Part print with two shaded views. Sizes in mm from the minimum x, y, z corner. A direction names the side the tool comes from. Round coordinates to 2 decimals unless told otherwise and drop trailing zeros. Write each loop counter-clockwise with the first axis right and the second up, starting at its lowest first coordinate (ties: lowest second). Pieces come first, ordered by that corner, then holes. Notation, with made-up numbers: (86, -22) -> (105, -22) arc R22 ccw to (105, 3) -> close; hole circle Ø11 at (15.5, -2.75). An arc over 180 degrees is marked (long way). Return JSON: item names as keys, results as strings. Group by question number.
(1) Tool access for the marked faces 1, 2 and 3: list every direction of +Z, -Z, +X, -X, +Y, -Y with a clear straight run to the whole face (end or side of a thin tool).
(2) Drill centre lines: L1, parallel to Z at x = 69.5, y = 12; L2, parallel to Y at x = 11, z = 58.5; L3, parallel to Y at x = 35, z = 49. Where is each one in solid material? Low to high. Write a range as from..to.
(3) Saw through at C-C (y = 36). List the corners of the cut face in (x, z), plus the area to 3 significant figures.
(4) Saw through at D-D (x = 66.5). List the corners of the cut face in (y, z), plus the area to 3 significant figures.
(5) Saw through at A-A (x = 35.5). List the corners of the cut face in (y, z).
(6) Drop flat-ended pins along their axis: pin 1 Ø1 at (x, y) = (72, 11) entering from -Z; pin 2 Ø2 at (x, z) = (35.5, 26) entering from -Y; pin 3 Ø1.2 at (y, z) = (76, 23) entering from -X; pin 4 Ø12 at (y, z) = (66.5, 60.5) entering from +X. Give the stop position or say it passes through.
(7) Saw through at B-B (z = 10). List the corners of the cut face in (x, y).
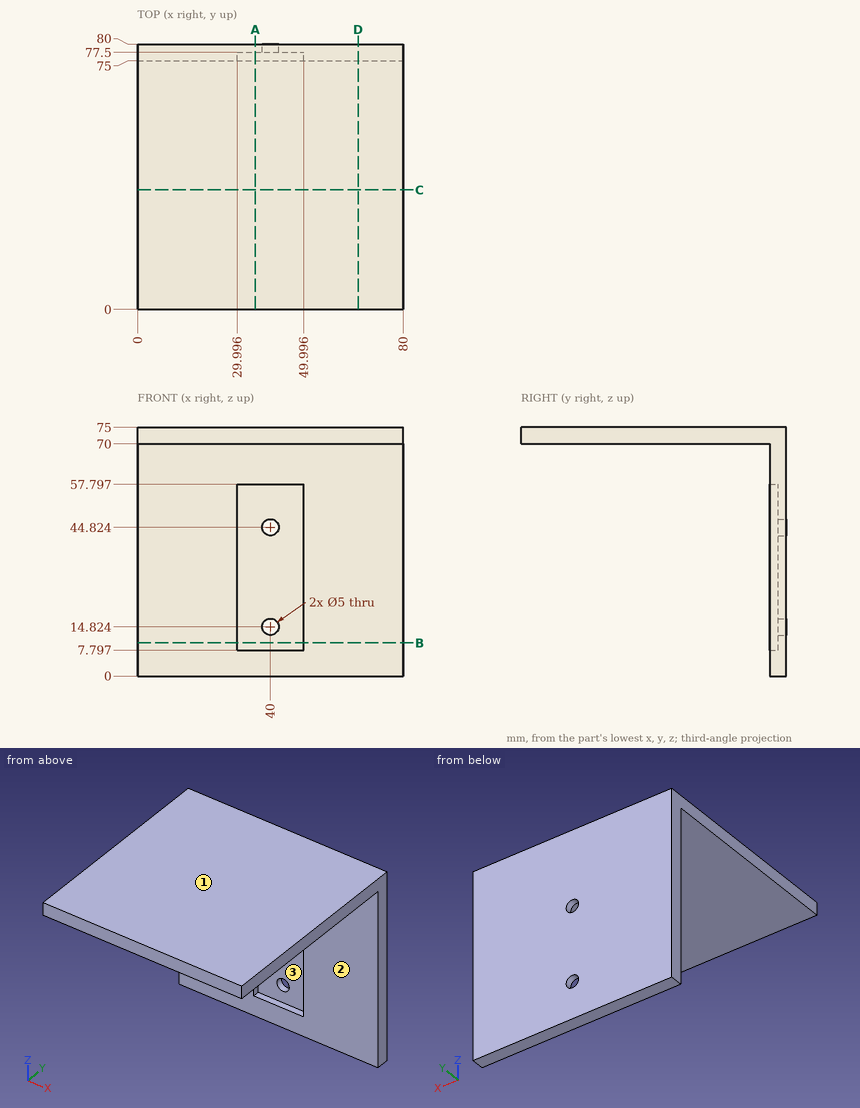
Computed values:
{
 "1": {"face 1": "+Z, +X, -X, +Y, -Y", "face 2": "-Z, +X, -X, -Y", "face 3": "-Y"},
 "2": {"L1": "70..75", "L2": "75..80", "L3": "77.5..80"},
 "3": {"outline": "(0, 70) -> (80, 70) -> (80, 75) -> (0, 75) -> close", "area": "400 mm2"},
 "4": {"outline": "(0, 70) -> (75, 70) -> (75, 0) -> (80, 0) -> (80, 75) -> (0, 75) -> close", "area": "750 mm2"},
 "5": {"outline": "(0, 70) -> (75, 70) -> (75, 57.8) -> (77.5, 57.8) -> (77.5, 7.8) -> (75, 7.8) -> (75, 0) -> (80, 0) -> (80, 75) -> (0, 75) -> close"},
 "6": {"pin 1": "z = 70", "pin 2": "y = 77.5", "pin 3": "x = 0", "pin 4": "through"},
 "7": {"outline": "(0, 75) -> (30, 75) -> (30, 77.5) -> (50, 77.5) -> (50, 75) -> (80, 75) -> (80, 80) -> (0, 80) -> close"}
}
